```python
from build123d import *

# Parameters (mm, degrees)
SKETCH1_W            = 224
SKETCH1_H            = 40
BOSS_EXTRUDE1_DEPTH  = 6
SKETCH2_W            = 6
SKETCH2_H            = 10
CUT_EXTRUDE1_DEPTH   = 228.622494495
LPATTERN1_COUNT      = 2
LPATTERN1_PITCH      = 206
LPATTERN1_COUNT_DIR2 = 2
LPATTERN1_PITCH_DIR2 = 30
SKETCH3_W            = 70
SKETCH3_H            = 6
CUT_EXTRUDE2_DEPTH   = 228.622494495
SKETCH4_W            = 130
SKETCH4_H            = 15
CUT_EXTRUDE3_DEPTH   = 10


with BuildPart() as part:
    # Sketch1 → Boss-Extrude1 (new body)
    with BuildSketch(Plane.XY):
        with Locations((-112, 20)):
            Rectangle(SKETCH1_W, SKETCH1_H)
    extrude(amount=BOSS_EXTRUDE1_DEPTH)

    # Sketch2 → Cut-Extrude1 (cut, through all)
    with BuildSketch(Plane.XY.offset(6)):
        with Locations((-215, 35)):
            Rectangle(SKETCH2_W, SKETCH2_H)
    cut_extrude1 = extrude(amount=-CUT_EXTRUDE1_DEPTH, mode=Mode.SUBTRACT)

    # LPattern1: Cut-Extrude1 2 × 2
    with Locations(*[(i * LPATTERN1_PITCH, -j * LPATTERN1_PITCH_DIR2, 0) for i in range(LPATTERN1_COUNT) for j in range(LPATTERN1_COUNT_DIR2) if (i, j) != (0, 0)]):
        add(cut_extrude1, mode=Mode.SUBTRACT)

    # Sketch3 → Cut-Extrude2 (cut, through all)
    with BuildSketch(Plane.XY.offset(6)):
        with Locations((-112, 37)):
            Rectangle(SKETCH3_W, SKETCH3_H)
    extrude(amount=-CUT_EXTRUDE2_DEPTH, mode=Mode.SUBTRACT)

    # Sketch4 → Cut-Extrude3 (cut)
    with BuildSketch(Plane.XY.offset(6)):
        with Locations((-112, 7.5)):
            Rectangle(SKETCH4_W, SKETCH4_H)
    extrude(amount=-CUT_EXTRUDE3_DEPTH, mode=Mode.SUBTRACT)


solid = part.part
```
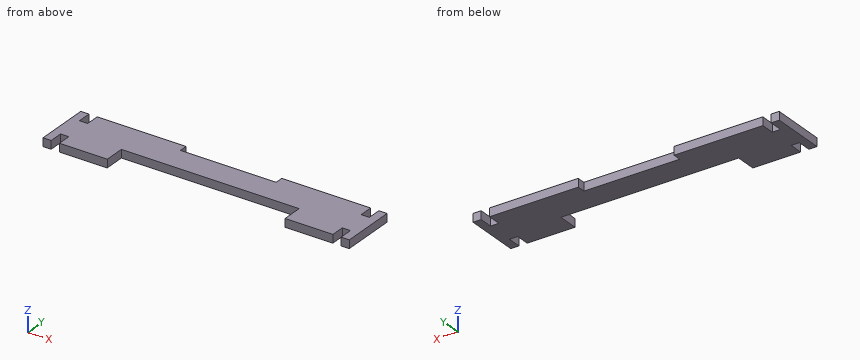
Input: part model. Units: mm. Frame: model coordinates. Coordinates: 2 decimals unless noted, no trailing zeros. Loops run counter-clockwise (first coordinate to the right, second up) from the corner with the lowest first, then second, coordinate; pieces in that order, holes last. Notation, with made-up numbers: M 30,49 L 79,49 A27 cw 79,69 Z; hole C 14,-25 d8. An arc over 180 degrees is marked long. Use a Markdown table: item, result. Add a question column.
1) Section A-A, the plane y = 6.5. Return the cut outline in (x, z), plus the area to 3 significant figures.
2) Pin query (flat end, axial travel): P1, Ø3, axis at x = -123, z = 2.5, coming from the +Y side; P2, Ø3, axis at x = -159.5, z = 1.5, coming from the -Y side; P3, Ø3, axis at x = -163.5, y = 12.5, coming from the -Z side. Return the tip coordinate at first contact, or that it passes through.
3) Section C-C, the plane x = -83. Return the cut outline in (y, z).
4) Section B-B, the plane z = 3.9. Return the cut outline in (x, y).
5) Line query: L1, parallel to X at y = 7, z = 5.7; L2, parallel to X at y = 34.5, z = 1.5; L3, parallel to X at y = 14.5, z = 1. Output: solid intervals per line, ascending. Write a range as from..to.
Answer below:
| question | item | result |
|---|---|---|
| 1 | outline | M -224,0 L -218,0 L -218,6 L -224,6 Z; M -212,0 L -177,0 L -177,6 L -212,6 Z; M -47,0 L -12,0 L -12,6 L -47,6 Z; M -6,0 L 0,0 L 0,6 L -6,6 Z |
| 1 | area | 492 mm2 |
| 2 | P1 | y = 34 |
| 2 | P2 | y = 15 |
| 2 | P3 | through |
| 3 | outline | M 15,0 L 34,0 L 34,6 L 15,6 Z |
| 4 | outline | M -224,0 L -218,0 L -218,10 L -212,10 L -212,0 L -177,0 L -177,15 L -47,15 L -47,0 L -12,0 L -12,10 L -6,10 L -6,0 L 0,0 L 0,40 L -6,40 L -6,30 L -12,30 L -12,40 L -77,40 L -77,34 L -147,34 L -147,40 L -212,40 L -212,30 L -218,30 L -218,40 L -224,40 Z |
| 5 | L1 | -224..-218, -212..-177, -47..-12, -6..0 |
| 5 | L2 | -224..-218, -212..-147, -77..-12, -6..0 |
| 5 | L3 | -224..-177, -47..0 |
